Here's how the part is built. I have some questions about the finished solid (model axes, mm). A direction names the side the tool comes from. Give positions to 0.01 mm unless a question says otherwise; leave off trailing zeros. Write each loop counter-clockwise with the first axis right and the second up, starting at its lowest first coordinate (ties: lowest second). Pieces come first, ordered by that corner, then holes. Notation, with made-up numbers: (9, 22) - (56, 22) arc R29 cw to (56, 45) - close; hole circle Ø8 at (-33, -29.5). An arc over 180 degrees is marked (long way). One line per item, written item: value. Start each with the question number.
1) Please list where these lines run through material, in increasing order: L1, parallel to Y at x = 40, z = 77; L2, parallel to Z at x = 40.5, y = 0; L3, parallel to Y at x = 0, z = 36.3. Write a range as [from, to].
2) Imagine slicing it at C-C on x = 58.5. Write out the boundary of the cut face in (y, z) (3 decimals), plus the area to 3 significant figures.
3) We'd pull the mould along Z, two halves only. Please class faces 4 (the cylindrical face through (7.262, -32.703, 36.479)), 5 (the flat face through (-14, 31, 35)), 6 (the flat face through (42, -31, 91)): +Z half, -Z half, draft (parallel to the pull), parting line (faces both ways), or undercut.
4) Imagine slicing it at A-A on y = 0. Count the separate pieces of the cut face and the enclosed holes in it, plus the area to 3 significant figures.
5) I'm going to push flat-ended pins straight in: P1, Ø12, axis at y = 8.5, z = 16, coming from the -X side; P2, Ø5, axis at y = 30, z = 12, coming from the -X side; P3, Ø6, axis at y = -31.5, z = 18, coming from the -X side. Where does each tip first touch, or does it pass through?
6) On a 3-axis mill with a long thin cutter (end or side, diameter ignored), from which of +Z, -Z, +X, -X, +Y, -Y can I reach the whole of each face in a straight line? I mean faces 1 (the conical face through (59.745, 23.139, 46.823)), 2 (the flat face through (39, 37, 75)), 3 (the conical face through (37.99, 1.67, 17.26)). Say none if no direction works.
7) Imagine slicing it at B-B on z = 23. Write out the boundary of the cut face in (x, y).
Autodesk Inventor part; units mm, degrees
ref_plane "YZ Plane" through (0, 0, 0) normal (1, 0, 0) x (0, 1, 0)
ref_plane "XZ Plane" through (0, 0, 0) normal (0, 1, 0) x (-1, 0, 0)
ref_plane "XY Plane" through (0, 0, 0) normal (0, 0, 1) x (1, 0, 0)
sketch "Sketch1" plane through (0, 0, 0) normal (0, 1, 0) x (-1, 0, 0)
  line L0 (0, 0) -> (0, 38)
  line L1 (41.2001, 0) -> (0, 0)
  line L2 (0, 38) -> (40.8201, 38)
  line L3 (37.85, 35) -> (38.2, 0)
  line L4 (41.2001, 0) -> (40.8201, 38)
  line L5 (33.5, 38) -> (33.5, 35)
  line L6 (33.5, 35) -> (37.85, 35)
  line L7 (33.5, 35) -> (0, 35) construction
  dimension "d0" = 76.4
  dimension "d3" = 75.7
  dimension "d4" = 3
  dimension "d5" = 35
  dimension "d6" = 3
  dimension "d7" = 67
revolve "Revolution1" add sketch "Sketch1" angle 360 about axis through (0, 0, 0) along (0, 0, 1) contours L3 L6 L5 L2 L4 L1
sketch "Sketch2" plane through (0, 0, 38) normal (0, 0, 1) x (1, 0, 0)
  circle A0 centre (0, 0) radius 40.8201
  circle A1 centre (0, 0) radius 33.5
  circle A2 centre (0, 0) radius 36.6
  circle A3 centre (0, 0) radius 33.5
  dimension "d8" = 67
  dimension "d9" = 3.1
sketch "Sketch3" plane through (0, 0, 0) normal (0, 1, 0) x (-1, 0, 0)
  arc A0 (0, 38) -> (-39, 77) centre (-39, 38) ccw
  dimension "d10" = 39
  dimension "d11" = 39
  dimension "d12" = 39
sweep "Sweep1" add profiles "Sketch2" path "Sketch3" contours A2
sketch "Sketch4" plane through (0, 0, 0) normal (0, 1, 0) x (-1, 0, 0)
  line L0 (-39, 43.5) -> (-39, 110.5)
  line L1 (-77, 77) -> (-39, 77)
  line L2 (-39, 77) -> (-39, 117.9202)
  line L3 (-39, 117.9202) -> (-77, 118.3002)
  line L4 (-77, 118.3002) -> (-77, 77)
  line L5 (-77, 115.2) -> (-42, 114.85)
  line L6 (-42, 117.9502) -> (-42, 110.5)
  line L7 (-42, 110.5) -> (-39, 110.5)
  line L8 (-42, 110.5) -> (-42, 77) construction
  dimension "d14" = 3.1
  dimension "d15" = 35
  dimension "d16" = 3
  dimension "d17" = 76.4
  dimension "d18" = 75.7
  dimension "d19" = 67
revolve "Revolution2" add sketch "Sketch4" angle 360 about axis through (77, 0, 77) along (-1, 0, 0) contours L7 L6 L3 L2 | L4 L3 L6 L5
equation "\"d0\" = d1"
equation "\"d3\" = d2"
equation "\"d4\" = t2"
equation "\"d5\" = l1"
equation "\"d6\" = t2"
equation "\"d7\" = d"
equation "\"d8\" = d"
equation "\"d9\" = t1"
equation "\"d10\" = Z - t2"
equation "\"d11\" = Z - t2"
equation "\"d12\" = Z - t2"
equation "\"d14\" = t1"
equation "\"d15\" = l1"
equation "\"d16\" = t2"
equation "\"d17\" = d1"
equation "\"d18\" = d2"
equation "\"d19\" = d"
equation "\"d\" = 67"
equation "\"d1\" = 76.4"
equation "\"d2\" = 75.7"
equation "\"l1\" = 35"
equation "\"L\" = 77"
equation "\"t1\" = 3.1"
equation "\"t2\" = 3"
equation "\"Z\" = 42"
properties part number "JIS K 6739 90 Deg Elbow (DL) 65" material "PVC, Unplasticized"
Numbers:
1. L1: [-40.93, -33.5], [33.5, 40.93]
1. L2: [0, 43.5], [110.5, 117.94]
1. L3: [-40.84, -33.5], [33.5, 40.84]
2. outline: circle Ø82.23 at (0, 77); hole circle Ø76.03 at (0, 77)
2. area: 771 mm^2
3. face 4: draft
3. face 5: -Z half
3. face 6: undercut
4. separate pieces: 2
4. enclosed holes: 1
4. area: 892 mm^2
5. P1: x = -40.97
5. P2: x = -30.52
5. P3: x = -29.5
6. face 1: +X
6. face 2: none
6. face 3: -Z
7. outline: circle Ø81.94 at (0, 0); hole circle Ø75.94 at (0, 0)
